Autodesk Inventor part; units mm, degrees
ref_plane "YZ Plane" through (0, 0, 0) normal (1, 0, 0) x (0, 1, 0)
ref_plane "XZ Plane" through (0, 0, 0) normal (0, 1, 0) x (-1, 0, 0)
ref_plane "XY Plane" through (0, 0, 0) normal (0, 0, 1) x (1, 0, 0)
sketch "Sketch1" plane through (0, 0, 0) normal (0, 0, 1) x (1, 0, 0)
  circle A0 centre (0, 0) radius 5
  dimension "d0" = 10
extrude "Extrusion1" add sketch "Sketch1" along normal blind 10
sketch "Sketch3" plane through (0, 0, 10) normal (0, 0, 1) x (1, 0, 0)
  circle A0 centre (0, 0) radius 5 construction
  arc A1 (-2, -4.5826) -> (-0.9, -7.4458) centre (12.4788, -0.663) ccw
  arc A2 (0.9, -7.4458) -> (2, -4.5826) centre (-12.4788, -0.663) ccw
  arc A3 (-2, -4.5826) -> (2, -4.5826) centre (0, 0) ccw
  arc A4 (-0.9, -7.4458) -> (0.9, -7.4458) centre (0, 12.5339) ccw
  circle A5 centre (0, 0) radius 7.5 construction
  line L0 (0, 0) -> (0, -8.6797) construction
  arc A6 (2.9686, -4.0233) -> (5.9983, -4.5023) centre (6.8136, 10.4755) ccw
  arc A7 (2.9686, -4.0233) -> (4.9686, -0.5592) centre (0, 0) ccw
  arc A8 (6.8983, -2.9435) -> (4.9686, -0.5592) centre (-5.6653, -11.1385) ccw
  arc A9 (5.9983, -4.5023) -> (6.8983, -2.9435) centre (-10.8547, 6.267) ccw
  arc A10 (4.9686, 0.5592) -> (6.8983, 2.9435) centre (-5.6653, 11.1385) ccw
  arc A11 (4.9686, 0.5592) -> (2.9686, 4.0233) centre (0, 0) ccw
  arc A12 (5.9983, 4.5023) -> (2.9686, 4.0233) centre (6.8136, -10.4755) ccw
  arc A13 (6.8983, 2.9435) -> (5.9983, 4.5023) centre (-10.8547, -6.267) ccw
  arc A14 (2, 4.5826) -> (0.9, 7.4458) centre (-12.4788, 0.663) ccw
  arc A15 (2, 4.5826) -> (-2, 4.5826) centre (0, 0) ccw
  arc A16 (-0.9, 7.4458) -> (-2, 4.5826) centre (12.4788, 0.663) ccw
  arc A17 (0.9, 7.4458) -> (-0.9, 7.4458) centre (0, -12.5339) ccw
  arc A18 (-2.9686, 4.0233) -> (-5.9983, 4.5023) centre (-6.8136, -10.4755) ccw
  arc A19 (-2.9686, 4.0233) -> (-4.9686, 0.5592) centre (0, 0) ccw
  arc A20 (-6.8983, 2.9435) -> (-4.9686, 0.5592) centre (5.6653, 11.1385) ccw
  arc A21 (-5.9983, 4.5023) -> (-6.8983, 2.9435) centre (10.8547, -6.267) ccw
  arc A22 (-4.9686, -0.5592) -> (-6.8983, -2.9435) centre (5.6653, -11.1385) ccw
  arc A23 (-4.9686, -0.5592) -> (-2.9686, -4.0233) centre (0, 0) ccw
  arc A24 (-5.9983, -4.5023) -> (-2.9686, -4.0233) centre (-6.8136, 10.4755) ccw
  arc A25 (-6.8983, -2.9435) -> (-5.9983, -4.5023) centre (10.8547, 6.267) ccw
  point P0 (0, -7.4661)
  point P1 (0, -5)
  point P2 (4.3301, -2.5)
  point P3 (6.4658, -3.733)
  point P4 (4.3301, 2.5)
  point P5 (6.4658, 3.733)
  point P6 (0, 5)
  point P7 (0, 7.4661)
  point P8 (-4.3301, 2.5)
  point P9 (-6.4658, 3.733)
  point P10 (-4.3301, -2.5)
  point P11 (-6.4658, -3.733)
  dimension "d12" = 15
  dimension "d13" = 15
  dimension "d14" = 1.8
  dimension "d15" = 4
  dimension "d16" = 20
  dimension "d17" = 15
  dimension "d20" = 360
extrude "Extrusion2" add sketch "Sketch3" against normal blind 10
properties part number "SJ012" material "ABS Plastic"
Geometry: final body of the model. Coordinates: model frame, mm. A direction names the side the tool comes from. Give positions to 0.01 mm unless a question says otherwise; leave off trailing zeros. Order: outer loops, then holes, each group sorted by start corner. A loop starts at its lowest first (then second) coordinate and runs counter-clockwise, first axis right, second up. Notation, with made-up numbers: (-2.5, 40) -> (55.5, 40) arc R16 ccw to (55.5, 49) -> close; hole circle Ø10 at (50, 33). An arc over 180 degrees is marked (long way). Answer as a JSON object with one key per item and string values.
Q1. Section B-B (z = 1.75). Output: boundary loops of the cut face in (x, y).
Entries:
{"outline": "(-6.9, -2.94) arc R19.99 ccw to (-6, -4.5) arc R15 ccw to (-2.97, -4.02) arc R5 ccw to (-2, -4.58) arc R15 ccw to (-0.9, -7.45) arc R20 ccw to (0.9, -7.45) arc R15 ccw to (2, -4.58) arc R5 ccw to (2.97, -4.02) arc R15 ccw to (6, -4.5) arc R20.01 ccw to (6.9, -2.94) arc R15 ccw to (4.97, -0.56) arc R5 ccw to (4.97, 0.56) arc R15 ccw to (6.9, 2.94) arc R19.99 ccw to (6, 4.5) arc R15 ccw to (2.97, 4.02) arc R5 ccw to (2, 4.58) arc R15 ccw to (0.9, 7.45) arc R20 ccw to (-0.9, 7.45) arc R15 ccw to (-2, 4.58) arc R5 ccw to (-2.97, 4.02) arc R15 ccw to (-6, 4.5) arc R20.01 ccw to (-6.9, 2.94) arc R15 ccw to (-4.97, 0.56) arc R5 ccw to (-4.97, -0.56) arc R15 ccw to start"}
Q2. First-contact query: pin 1 (1.5 mm diameter, centred on x = -5, z = 7.5, fed in from +Y); pin 2 (2 mm diameter, centred on y = 0, z = 6, fed in from -X). Flat tips, straight axial feed; report the tip coordinate or a pass-through.
Entries:
{"pin 1": "stops at y = 4.49", "pin 2": "stops at x = -5.39"}
Q3. Material intervals for probe 1 along Y at (x, z) = (5.75, 9); probe 2 along Y at (x, z) = (0.75, 2.5); probe 3 along X at (y, z) = (6.25, 8.75), sorted ascending.
Entries:
{"probe 1": "y = -4.49 to -1.41, 1.41 to 4.49", "probe 2": "y = -7.45 to 7.45", "probe 3": "x = -1.44 to 1.44"}
Q4. Section D-D (x = -1.5). Output: boundary loops of the cut face in (y, z), plus the area to 3 significant figures.
Entries:
{"outline": "(-6.1, 0) -> (6.1, 0) -> (6.1, 10) -> (-6.1, 10) -> close", "area": "122 mm^2"}
Q5. Access query for faces 5 (the cylindrical face through (-5, 0, 5)), 6 (the cylindrical face through (6.01, -1.72, 5.07)), 7 (the cylindrical face through (6.46, -3.74, 5.07)), 8 (the cylindrical face through (-4.492, -4.344, 5.07)), 9 (the cylindrical face through (-2.507, 4.326, 4.93)). Directions: +Z, -Z, +X, -X, +Y, -Y. A direction counts if a zero-diameter tool reaches every point of the face in a straight line with its end or side. Return the directions, or none.
Entries:
{"face 5": "+Z, -Z, -X", "face 6": "+Z, -Z, +X", "face 7": "+Z, -Z, +X, -Y", "face 8": "+Z, -Z, -Y", "face 9": "+Z, -Z, +Y"}
Q6. Section C-C (y = -0.25). Output: boundary loops of the cut face in (x, z), plus the area to 3 significant figures.
Entries:
{"outline": "(-4.99, 0) -> (4.99, 0) -> (4.99, 10) -> (-4.99, 10) -> close", "area": "99.9 mm^2"}
Q7. Draft query along Y for faces 1 (the cylindrical face through (5, 0, 5)), 2 (the cylindrical face through (1.53, 6.02, 5.07)), 3 (the cylindrical face through (2.507, -4.326, 4.93)), 4 (the flat face through (0, 0, 10)). Return one class per face: released by +Y, released by -Y, zero draft, split by the parting line, or undercut.
Entries:
{"face 1": "undercut", "face 2": "released by +Y", "face 3": "released by -Y", "face 4": "zero draft"}
Q8. Section A-A (y = -4.25). Output: boundary loops of the cut face in (x, z), plus the area to 3 significant figures.
Entries:
{"outline": "(-6.16, 0) -> (-3.96, 0) -> (-3.96, 10) -> (-6.16, 10) -> close; (-2.63, 0) -> (2.63, 0) -> (2.63, 10) -> (-2.63, 10) -> close; (3.96, 0) -> (6.16, 0) -> (6.16, 10) -> (3.96, 10) -> close", "area": "96.7 mm^2"}
